Autodesk Inventor part; units mm, degrees
ref_plane "YZ Plane" through (0, 0, 0) normal (1, 0, 0) x (0, 1, 0)
ref_plane "XZ Plane" through (0, 0, 0) normal (0, 1, 0) x (-1, 0, 0)
ref_plane "XY Plane" through (0, 0, 0) normal (0, 0, 1) x (1, 0, 0)
sketch "Szkic1" plane through (0, 0, 0) normal (0, 1, 0) x (-1, 0, 0)
  point P0 (0, 0)
sketch "Szkic2" plane through (0, 0, 0) normal (0, 1, 0) x (-1, 0, 0)
  line L0 (60, -30) -> (-60, -30)
  line L1 (-60, -30) -> (-60, 30)
  line L2 (-60, 30) -> (60, 30)
  line L3 (60, 30) -> (60, -30)
  line L4 (60, -30) -> (-60, 30) construction
  line L5 (-60, -30) -> (60, 30) construction
  point P0 (0, 0)
  dimension "d0" = 120
  dimension "d1" = 60
extrude "Wyciągnięcie proste1" add sketch "Szkic2" along normal blind 10
sketch "Szkic3" plane through (0, 10, 0) normal (0, 1, 0) x (1, 0, 0)
  line L0 (0, 0) -> (50, 0)
  line L1 (60, -30) -> (60, 30)
  line L2 (50, 0) -> (60, 0)
  line L3 (60, 0) -> (60, 15)
  line L4 (60, 15) -> (50, 15)
  line L5 (50, 15) -> (50, 0)
  dimension "d4" = 50
  dimension "d5" = 15
extrude "Wyciągnięcie proste2" cut sketch "Szkic3" against normal blind 10
mirror "Odbij1" about plane through (0, 0, 0) normal (0, 0, 1) of "Wyciągnięcie proste2"
mirror "Odbij2" about plane through (0, 0, 0) normal (1, 0, 0) of "Wyciągnięcie proste2"
mirror "Odbij3" about plane through (0, 0, 0) normal (0, 0, 1) of "Wyciągnięcie proste2", "Odbij2"
sketch "Szkic4" plane through (0, 10, 0) normal (0, 1, 0) x (1, 0, 0)
  line L0 (-50, 15) -> (50, 15)
  line L1 (50, 15) -> (50, -15)
  line L2 (50, -15) -> (-50, -15)
  line L3 (-50, -15) -> (-50, 15)
  line L4 (-50, 15) -> (50, -15) construction
  line L5 (50, 15) -> (-50, -15) construction
  point P0 (0, 0)
extrude "Wyciągnięcie proste3" cut sketch "Szkic4" against normal blind 2
sketch "Szkic5" plane through (0, 10, 0) normal (0, 1, 0) x (1, 0, 0)
  line L0 (0, 0) -> (0, -16)
  line L1 (50, -15) -> (-50, -15)
  line L2 (0, 0) -> (16, 0) construction
  line L3 (-6, -15) -> (6, -15)
  line L4 (6, -15) -> (6, -17)
  line L5 (6, -17) -> (-6, -17)
  line L6 (-6, -17) -> (-6, -15)
  line L7 (-6, -15) -> (6, -17) construction
  line L8 (6, -15) -> (-6, -17) construction
  dimension "d10" = 16
  dimension "d11" = 90
  dimension "d12" = 12
  dimension "d13" = 2
extrude "Wyciągnięcie proste4" add sketch "Szkic5" along normal blind 20
sketch "Szkic6" plane through (-6, 10, 17) normal (0, 0, 1) x (1, 0, 0)
  point P0 (6, -10)
sketch "Szkic7" plane through (-6, 10, 17) normal (0, 0, 1) x (1, 0, 0)
  line L0 (12, 20) -> (0, 20)
  line L1 (6, 20) -> (6, 14)
  line L2 (6, 20) -> (12, 20) construction
  circle A0 centre (6, 14) radius 4
  point P0 (6, -10)
  dimension "d16" = 6
  dimension "d17" = 90
  dimension "d18" = 8
extrude "Wyciągnięcie proste5" cut sketch "Szkic7" against normal through all
sketch "Szkic8" plane through (0, 10, 0) normal (0, 1, 0) x (1, 0, 0)
  point P0 (0, 0)
mirror "Odbij4" about plane through (0, 0, 0) normal (0, 0, 1) of "Wyciągnięcie proste4", "Wyciągnięcie proste5"
sketch "Szkic9" plane through (0, 10, 0) normal (0, 1, 0) x (1, 0, 0)
  line L0 (6, 15) -> (60, 15)
  line L1 (60, 15) -> (45, 15)
  line L2 (45, 15) -> (45, 16.2)
  line L3 (45, 16.2) -> (60, 16.2)
  line L4 (60, 16.2) -> (60, 15)
  point P0 (0, 0)
  dimension "d21" = 15
  dimension "d22" = 1.2
extrude "Wyciągnięcie proste6" add sketch "Szkic9" along normal blind 5
mirror "Odbij5" about plane through (0, 0, 0) normal (1, 0, 0) of "Wyciągnięcie proste6"
mirror "Odbij6" about plane through (0, 0, 0) normal (0, 0, 1) of "Wyciągnięcie proste6"
sketch "Szkic10" plane through (0, 10, 0) normal (0, 1, 0) x (1, 0, 0)
  line L0 (60, 30) -> (-60, 30)
  line L1 (60, 15) -> (60, 30)
  line L2 (-60, 30) -> (60, 30)
  line L3 (60, 30) -> (60, 28.8)
  line L4 (60, 28.8) -> (-60, 28.8)
  line L5 (-60, 28.8) -> (-60, 30)
  point P0 (0, 0)
  dimension "d25" = 1.2
extrude "Wyciągnięcie proste7" cut sketch "Szkic10" against normal blind 4
mirror "Odbij7" about plane through (0, 0, 0) normal (0, 0, 1) of "Wyciągnięcie proste7"
sketch "Szkic11" plane through (0, 10, 0) normal (0, 1, 0) x (1, 0, 0)
  point P0 (0, 0)
sketch "Szkic12" plane through (0, 15, 0) normal (0, 1, 0) x (1, 0, 0)
  line L0 (60, 28.8) -> (-60, 28.8)
  line L1 (-60, -28.8) -> (60, -28.8)
  line L2 (60, 28.8) -> (58.8, 28.8)
  line L3 (58.8, 28.8) -> (58.8, -28.8)
  line L4 (58.8, -28.8) -> (60, -28.8)
  line L5 (60, -28.8) -> (60, 28.8)
  point P0 (0, 0)
  dimension "d28" = 1.2
extrude "Wyciągnięcie proste8" cut sketch "Szkic12" against normal up to surface (9 mm away)
mirror "Odbij8" about plane through (0, 0, 0) normal (1, 0, 0) of "Wyciągnięcie proste8"
sketch "Szkic13" plane through (0, 0, 0) normal (0, -1, 0) x (1, 0, 0)
  line L0 (60, -30) -> (-60, -30)
  line L1 (60, -30) -> (-60, -30)
  line L2 (-60, -30) -> (-60, 30)
  line L3 (-60, 30) -> (60, 30)
  line L4 (60, 30) -> (60, -30)
  point P0 (0, 0)
extrude "Wyciągnięcie proste9" cut sketch "Szkic13" against normal blind 4
mirror "Odbij9" about plane through (0, 0, 0) normal (0, 0, 1) of "Wyciągnięcie proste6", "Odbij5"
sketch "Szkic14" plane through (-60, 10, 15) normal (-1, 0, 0) x (0, 0, 1)
  line L0 (1.2, 0) -> (1.2, 5)
  line L1 (0, 0) -> (0, 20)
  line L2 (1.2, 5) -> (0, 5)
  line L3 (0, 5) -> (0, 0)
  line L4 (0, 0) -> (1.2, 0)
  line L5 (1.2, 0) -> (1.2, 5)
  point P0 (-15, -10)
extrude "Wyciągnięcie proste10" cut sketch "Szkic14" against normal up to surface (1.2 mm away)
sketch "Szkic15" plane through (58.8, 10, 15) normal (0, -1, 0) x (1, 0, 0)
  line L0 (1.2, 1.2) -> (-13.8, 1.2)
  line L1 (0, 0) -> (1.2, 0)
  line L2 (1.2, 0) -> (1.2, 1.2)
  line L3 (1.2, 1.2) -> (0, 1.2)
  line L4 (0, 1.2) -> (0, 0)
  point P0 (-58.8, -15)
extrude "Wyciągnięcie proste11" cut sketch "Szkic15" against normal blind 10
properties part number "podstawka_pelna"
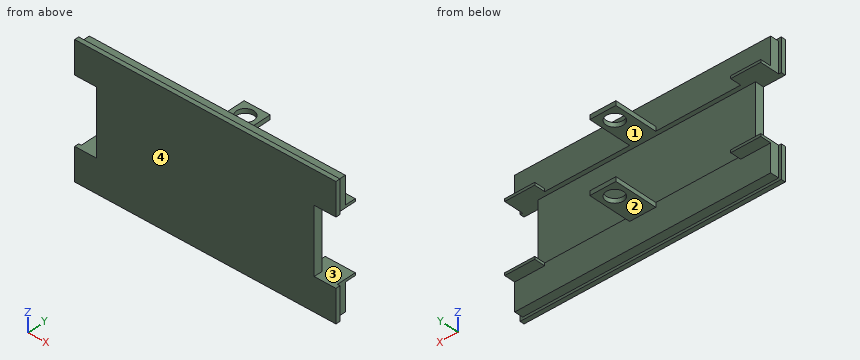
Design review of the part built by this model. Coordinates are the model's own, in mm. Face numbers are marked on the shaded views. Coordinates: 2 decimals unless noted, no trailing zeros. Order: outer loops, then holes, each group sorted by start corner. A loop starts at its lowest first (then second) coordinate and runs counter-clockwise, first axis right, second up. Notation, with made-up numbers: M 32,46 L 48,46 A3 cw 48,51 Z; hole C 56,-35.5 d10. An arc over 180 degrees is marked long. Answer as a JSON object with one key per item and string values. Group by question number.
1) Add section C-C, the plane x = 0. Write out the cut boundary in (y, z), then the cut area to 3 significant figures.
2) Add section B-B, the plane y = 24. Write out the cut boundary in (x, z), then the cut area to 3 significant figures.
3) Add section A-A, the plane y = 13.25. Write out the cut boundary in (x, z), then the cut area to 3 significant figures.
4) Wall thickness on L1, parallel to X at y = 24, z = -15.75; L2, parallel to Y at x = 0, z = 16.5; L3, parallel to Y at x = -22, z = 11: over which ranges is each line inside the solid? List them lowest first.
5) Add section D-D, the plane x = 12.5. Write out the cut boundary in (y, z).
6) For pin 1 (11 mm diameter, centred on x = 18, z = 23.5, fed in from +Y); pin 2 (3.5 mm diameter, centred on x = -2.5, y = 23.5, fed in from -Z); pin 3 (0.6 mm diameter, centred on x = -49.5, z = 15.5, fed in from +Y), all flat-tipped, find the tip position at first contact; note any pin that passes through.
7) Mouldability with a two-part tool opening along Z and no side actions: class the marked faces 1, 2, 3 and 4 as pulls with the +Z half, pulls with the -Z half, needs draft (parallel to the pull), parting line crosses it, or undercut.
Computed values:
{
 "1": {"outline": "M 4,-30 L 6,-30 L 6,-28.8 L 10,-28.8 L 10,-17 L 20,-17 L 20,-15 L 8,-15 L 8,15 L 20,15 L 20,17 L 10,17 L 10,28.8 L 6,28.8 L 6,30 L 4,30 Z; M 28,-17 L 30,-17 L 30,-15 L 28,-15 Z; M 28,15 L 30,15 L 30,17 L 28,17 Z", "area": "338 mm^2"},
 "2": {"outline": "M -6,-17 L -4,-17 L -4,-15 L -6,-15 Z; M -6,15 L -4,15 L -4,17 L -6,17 Z; M 4,-17 L 6,-17 L 6,-15 L 4,-15 Z; M 4,15 L 6,15 L 6,17 L 4,17 Z", "area": "16.0 mm^2"},
 "3": {"outline": "M -58.8,-16.2 L -45,-16.2 L -45,-15 L -58.8,-15 Z; M -58.8,15 L -45,15 L -45,16.2 L -58.8,16.2 Z; M -6,-17 L 6,-17 L 6,-15 L -6,-15 Z; M -6,15 L 6,15 L 6,17 L -6,17 Z; M 45,-16.2 L 58.8,-16.2 L 58.8,-15 L 45,-15 Z; M 45,15 L 58.8,15 L 58.8,16.2 L 45,16.2 Z", "area": "114 mm^2"},
 "4": {"L1": "x = -6 to -4, 4 to 6", "L2": "y = 4 to 20, 28 to 30", "L3": "y = 4 to 8"},
 "5": {"outline": "M 4,-30 L 6,-30 L 6,-28.8 L 10,-28.8 L 10,-15 L 8,-15 L 8,15 L 10,15 L 10,28.8 L 6,28.8 L 6,30 L 4,30 Z"},
 "6": {"pin 1": "stops at y = 10", "pin 2": "stops at z = -17", "pin 3": "stops at y = 15"},
 "7": {"face 1": "undercut", "face 2": "pulls with the -Z half", "face 3": "undercut", "face 4": "needs draft"}
}
